```python
from build123d import *

# Parameters (mm, degrees)
F1_DEPTH = 5
F3_DEPTH = 1000
F4_R     = 0.5
F5_DEPTH = 25
F6_W     = 75
F6_H     = 41
F7_DEPTH = 2.75


with BuildPart() as f1:
    # F0 (on Top) → F1 (new body)
    with BuildSketch(Plane.XY):
        with BuildLine():
            Line((0, 41), (0, 0))
            Line((0, 0), (80, 0))
            Line((80, 0), (80, 5))
            ThreePointArc((80, 5), (39.428626, 16.601304), (5, 41))
            Line((5, 41), (0, 41))
        make_face()
    extrude(amount=F1_DEPTH)

    # F2 (on face) → F3 (cut)
    with BuildSketch(Plane(origin=(0, 0, 0), x_dir=(0, -1, 0), z_dir=(-1, 0, 0))):
        with BuildLine():
            Line((-41, 2.75), (-41, 2.25))
            Line((-41, 2.25), (-3, 2.25))
            ThreePointArc((-3, 2.25), (-2.75, 2.5), (-3, 2.75))
            Line((-3, 2.75), (-41, 2.75))
        make_face()
    extrude(amount=-F3_DEPTH, mode=Mode.SUBTRACT)

    # F4 (on face) → F5 (cut)
    with BuildSketch(Plane(origin=(0, 0, 0), x_dir=(0, -1, 0), z_dir=(-1, 0, 0))):
        with Locations((-40.3, 2.5)):
            Circle(F4_R)
    extrude(amount=-F5_DEPTH, mode=Mode.SUBTRACT)

    # F6 (on face) → F7 (cut)
    with BuildSketch(Plane.XY.offset(5)):
        with Locations((42.5, 20.5)):
            Rectangle(F6_W, F6_H)
    extrude(amount=-F7_DEPTH, mode=Mode.SUBTRACT)


solid = f1.part
```
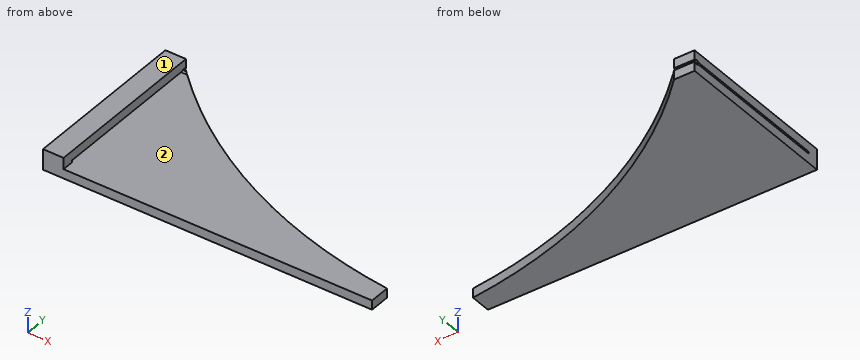
Source: CAD feature listing. Evaluate the final solid. Frame: model axes, mm. Face numbers are marked on the shaded views. A direction names the side the tool comes from. Coordinates: 2 decimals unless noted, no trailing zeros. Loops run counter-clockwise (first coordinate to the right, second up) from the corner with the lowest first, then second, coordinate; pieces in that order, holes last. Notation, with made-up numbers: M -20.5,88.25 L 3.5,88.25 A21 ccw 3.5,104.25 Z; hole C 48.25,85 d11. An arc over 180 degrees is marked long. Put each result on its own line as item: value. Start each with the question number.
1) Contact query for flat-ended pins moving along their axis: pin 1 Ø2 at (x, z) = (58.5, 3) entering from +Y; pin 2 Ø10 at (x, y) = (43.5, 18.5) entering from +Z. Output: stop coordinate, or through.
2) Ray query, L1, parallel to Z at x = 4.5, y = 13.5; L2, parallel to Z at x = 27, y = 22; L3, parallel to X at y = 28.5, z = 2.95. Return the intervals inside material, ascending. Write a range as from..to.
3) Cut plane C-C on x = 26. Return the cut outline in (y, z), then the cut area to 3 significant figures.
4) Reachability of the marked faces 1 and 2 from +Z, -Z, +X, -X, +Y, -Y: full face, straight path, thin tool, end or side. Return the list, or none.
5) Cut plane A-A on y = 8. Return the cut outline in (x, z).
6) Cut plane D-D on x = 35.5. Return the cut outline in (y, z).
7) Cut plane B-B on y = 35.5. Return the cut outline in (x, z), then the cut area to 3 significant figures.
The answers:
1. pin 1: stops at y = 9.49
1. pin 2: stops at z = 2.25
2. L1: z = 0..2.25, 2.75..5
2. L2: z = 0..2.25
2. L3: x = 0..5
3. outline: M 0,0 L 24.09,0 L 24.09,2.25 L 0,2.25 Z
3. area: 54.2 mm²
4. face 1: +Z, +X, -X, +Y, -Y
4. face 2: +X, +Y
5. outline: M 0,0 L 63.26,0 L 63.26,2.25 L 0,2.25 Z; M 0,2.75 L 5,2.75 L 5,5 L 0,5 Z
6. outline: M 0,0 L 18.57,0 L 18.57,2.25 L 0,2.25 Z
7. outline: M 0,0 L 10.86,0 L 10.86,2.25 L 0,2.25 Z; M 0,2.75 L 5,2.75 L 5,5 L 0,5 Z
7. area: 35.7 mm²
